Part model, mm, in its own coordinate system. Give positions to 0.01 mm unless a question says otherwise; leave off trailing zeros. Loops run counter-clockwise (first coordinate to the right, second up) from the corner with the lowest first, then second, coordinate; pieces in that order, holes last. Notation, with made-up numbers: (30.5, 69) -> (50.5, 69) arc R23 cw to (50.5, 100) -> close; hole circle Ø8 at (-34.75, -20.5). An arc over 180 degrees is marked (long way). One line per question, with ' | ' between items.
```python
from build123d import *

# Parameters (mm, degrees)
F1_DEPTH = 1


# Not quite as in the source:
# - a feature names something its author has since deleted; it is built from what else it names


with BuildPart() as f1:
    # F0 (on Right) → F1 (new body)
    with BuildSketch(Plane.YZ):
        Polygon((0, 0.75), (0, 0), (0, -0.25), (11.5, -0.25), (11.5, 0), (11.5, 0.75), (11.25, 0.75), (6.25, 0.75), (6.25, 1.25), (11.25, 1.25), (11.5, 1.25), (11.5, 2.25), (11.25, 2.25), (6.25, 2.25), (6.25, 2.75), (11.25, 2.75), (11.5, 2.75), (11.5, 3.75), (11.25, 3.75), (6.25, 3.75), (6.25, 4.25), (11.25, 4.25), (11.5, 4.25), (11.5, 5.25), (11.25, 5.25), (6.25, 5.25), (6.25, 5.75), (11.25, 5.75), (11.5, 5.75), (11.5, 6.75), (11.25, 6.75), (6.25, 6.75), (6.25, 7.25), (11.25, 7.25), (11.5, 7.25), (11.5, 8.25), (11.25, 8.25), (6.25, 8.25), (6.25, 8.75), (11.25, 8.75), (11.5, 8.75), (11.5, 9.75), (11.25, 9.75), (6.25, 9.75), (6.25, 10.25), (11.25, 10.25), (11.5, 10.25), (11.5, 11.25), (10.4177193716, 11.25), (10.4177193716, 15.3758693486), (9.0160202235, 15.3758693486), (9.0160202235, 11.25), (0, 11.25), (0, 10.25), (0.25, 10.25), (5.25, 10.25), (5.25, 9.75), (0.25, 9.75), (0, 9.75), (0, 8.75), (0.25, 8.75), (5.25, 8.75), (5.25, 8.25), (0.25, 8.25), (0, 8.25), (0, 7.25), (0.25, 7.25), (5.25, 7.25), (5.25, 6.75), (0.25, 6.75), (0, 6.75), (0, 5.75), (0.25, 5.75), (5.25, 5.75), (5.25, 5.25), (0.25, 5.25), (0, 5.25), (0, 4.25), (0.25, 4.25), (5.25, 4.25), (5.25, 3.75), (0.25, 3.75), (0, 3.75), (0, 2.75), (0.25, 2.75), (5.25, 2.75), (5.25, 2.25), (0.25, 2.25), (0, 2.25), (0, 1.25), (0.25, 1.25), (5.25, 1.25), (5.25, 0.75), (0.25, 0.75), align=None)
    extrude(amount=F1_DEPTH)


solid = f1.part
```
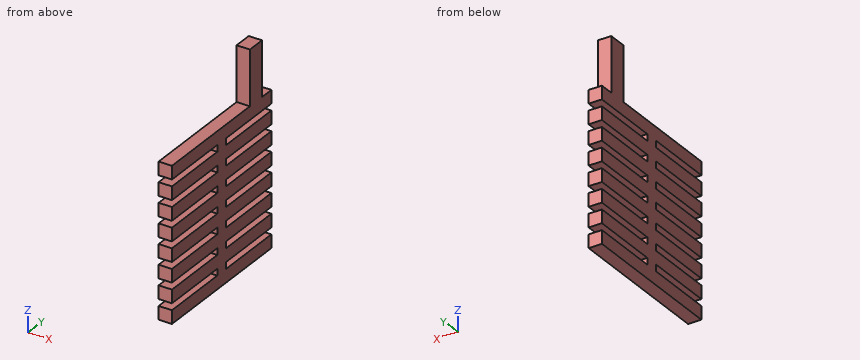
1) Saw through at A-A (y = 3.5). State how many separate pieces and enclosed holes the cut face has, and give its area (3 significant figures).
Found:
separate pieces: 8 | enclosed holes: 0 | area: 8.00 mm2
2) Pin check, flat tip, straight feed: P1, Ø0.6, axis at x = 0.5, z = 1, coming from the -Y side. Stop position of the tip, or through.
Found:
P1: y = 0
3) Drill centre lines: line 1 (Y direction, x = 0.4, z = 13.5); line 2 (Z direction, x = 0.5, y = 5.75); line 3 (Y direction, x = 0.45, z = 1). Where is each one in solid material? Low to high.
Found:
line 1: 9.02 to 10.42 | line 2: -0.25 to 11.25 | line 3: 5.25 to 6.25
4) Saw through at B-B (z = 13). Give the cut face in (x, y).
Found:
outline: (0, 9.02) -> (1, 9.02) -> (1, 10.42) -> (0, 10.42) -> close
